Check sheet for the modelled part. Datum: model origin and axes. Units: mm. A direction names the side the tool comes from. Coordinates: 2 decimals unless noted, no trailing zeros. Loops run counter-clockwise (first coordinate to the right, second up) from the corner with the lowest first, then second, coordinate; pieces in that order, holes last. Notation, with made-up numbers: M 39.25,-37.5 L 67.25,-37.5 A30 ccw 67.25,-14.5 Z; hole C 80.25,56 d1. An arc over 180 degrees is marked long. Answer in a Markdown table with one row per item. Add a question column.
```python
from build123d import *

# Parameters (mm, degrees)
POSICIONAMENTOS_R               = 8.2157
BASE_DEPTH                      = 3
FURO_DE_DI_METRO_2_6_2_6_1_D    = 2.6
BASE_DENTE_DEPTH                = 3
RAIO_DENTE_R                    = 1.342367201
PADR_OCIRCULAR1_COUNT           = 8
RAIO_DENTE_OF_PADR_OCIRCULAR1_R = 1.342367201
FURO_DE_DI_METRO_3_0_3_1_D      = 3
CORTE_EXTRUS_O1_DEPTH           = 21.724381776


with BuildPart() as part:
    # Posicionamentos → Base (new body)
    with BuildSketch(Plane.XY):
        Circle(POSICIONAMENTOS_R)
    extrude(amount=BASE_DEPTH)

    # Furo de diâmetro Ø2.6 (2.6)1 (through all)
    with Locations(Plane.XY.offset(3)):
        with Locations((0, 6.5), (-6.5, 0)):
            Hole(FURO_DE_DI_METRO_2_6_2_6_1_D / 2)

    # Dente → Base Dente (add, through all)
    with BuildSketch(Plane.XY):
        with BuildLine():
            Line((2.358922349, 10.642131153), (1.777928991, 8.021015833))
            ThreePointArc((1.777928991, 8.021015833), (0, 8.2157), (-1.777928991, 8.021015833))
            Line((-1.777928991, 8.021015833), (-2.358922349, 10.642131153))
            ThreePointArc((-2.358922349, 10.642131153), (-2.364262787, 11.016570047), (-2.263047735, 11.377109253))
            ThreePointArc((-2.263047735, 11.377109253), (-1.685191659, 13.049606095), (-0.650923694, 14.48538223))
            ThreePointArc((-0.650923694, 14.48538223), (0, 14.5), (0.650923694, 14.48538223))
            ThreePointArc((0.650923694, 14.48538223), (1.685191659, 13.049606095), (2.263047735, 11.377109253))
            ThreePointArc((2.263047735, 11.377109253), (2.364262787, 11.016570047), (2.358922349, 10.642131153))
        make_face()
    base_dente = extrude(amount=BASE_DENTE_DEPTH)

    # Raio Dente
    raio_dente_edges = [part.edges().sort_by_distance(p)[0] for p in [
        (-1.777928991, 8.021015833, 1.5),
        (1.777928991, 8.021015833, 1.5),
    ]]
    fillet(raio_dente_edges, radius=RAIO_DENTE_R)

    # PadrãoCircular1: Base Dente ×8 about axis
    padr_ocircular1_axis = Axis((0, 0, 0), (0, 0, 1))
    for i in range(1, PADR_OCIRCULAR1_COUNT):
        add(base_dente.rotate(padr_ocircular1_axis, i * 360 / PADR_OCIRCULAR1_COUNT))

    # Raio Dente of PadrãoCircular1
    raio_dente_of_padr_ocircular1_edges = [part.edges().sort_by_distance(p)[0] for p in [
        (-6.928900334, 4.414529041, 1.5),
        (-4.414529041, 6.928900334, 1.5),
        (-8.021015833, -1.777928991, 1.5),
        (-8.021015833, 1.777928991, 1.5),
        (-4.414529041, -6.928900334, 1.5),
        (-6.928900334, -4.414529041, 1.5),
        (1.777928991, -8.021015833, 1.5),
        (-1.777928991, -8.021015833, 1.5),
        (6.928900334, -4.414529041, 1.5),
        (4.414529041, -6.928900334, 1.5),
        (8.021015833, 1.777928991, 1.5),
        (8.021015833, -1.777928991, 1.5),
        (4.414529041, 6.928900334, 1.5),
        (6.928900334, 4.414529041, 1.5),
    ]]
    fillet(raio_dente_of_padr_ocircular1_edges, radius=RAIO_DENTE_OF_PADR_OCIRCULAR1_R)

    # Furo de diâmetro Ø3.0 (3)1 (through all)
    with Locations(Plane.XY.offset(3)):
        with Locations((0, 0)):
            Hole(FURO_DE_DI_METRO_3_0_3_1_D / 2)

    # Encaixe → Corte-extrusão1 (cut, through all)
    with BuildSketch(Plane.XY):
        with BuildLine():
            Line((-4, 0), (-4, -13.937359865))
            ThreePointArc((-4, -13.937359865), (10.253048327, -10.253048327), (13.937359865, 4))
            Line((13.937359865, 4), (0, 4))
            ThreePointArc((0, 4), (-2.828427125, 2.828427125), (-4, 0))
        make_face()
    extrude(amount=CORTE_EXTRUS_O1_DEPTH, mode=Mode.SUBTRACT)


solid = part.part
```
Q1. Mould release check, pull along X, two halves, no side actions. Record for faces 1 (the face through (-4, 3, 0)), 2 (the face through (-4.32, 7.41, 1.52)), 3 (the face through (-10.247, -10.259, 1.479)), 4 (the face through (-8.01, -10.41, 1.48)): released by +X, released by -X, zero draft, split by the parting line, or undercut.
Q2. Cross-section at B-B (y = -4.75). Record the cut outline in (x, z).
Q3. Thickness scan on L1, parallel to Y at x = 0, z = 0.95; L2, parallel to X at y = 9.75, z = 1.9. Record the ranges inside material, lowest first.
Q4. Go/stop test with flat-tipped pins: pin 1 (1 mm diameter, centred on y = 7, z = 1, fed in from +X); pin 2 (1.5 mm diameter, centred on y = 9.5, z = 1.5, fed in from -X); pin 3 (2.5 mm diameter, centred on x = -6.5, y = 0, fed in from -Z). Record where each tip stops, or that it passes through.
Q5. Cross-section at A-A (z = 2.65). Count the separate pieces of the cut face and the enclosed holes in it, plus the area to 3 significant figures.
Q6. Access from +Z, -Z, +X, -X, +Y, -Y to the whole of each face (thin tool, end or side, straight path). Record for faces 5 (the face through (8.01, 10.41, 1.48)), 6 (the face through (-8.321, -2.172, 1.521)), 7 (the face through (-10.427, -8.06, 1.479)).
Answer key:
| question | item | result |
|---|---|---|
| 1 | face 1 | zero draft |
| 1 | face 2 | undercut |
| 1 | face 3 | released by -X |
| 1 | face 4 | released by +X |
| 2 | outline | M -7.62,0 L -4,0 L -4,3 L -7.62,3 Z |
| 3 | L1 | 4 to 5.2, 7.8 to 14.5 |
| 3 | L2 | -10.7 to -6.6, -2.16 to 2.16, 6.6 to 10.7 |
| 4 | pin 1 | x = 10.22 |
| 4 | pin 2 | x = -10.7 |
| 4 | pin 3 | through |
| 5 | separate pieces | 1 |
| 5 | enclosed holes | 2 |
| 5 | area | 196 mm^2 |
| 6 | face 5 | +Z, -Z, +Y |
| 6 | face 6 | +Z, -Z |
| 6 | face 7 | +Z, -Z, -X |
